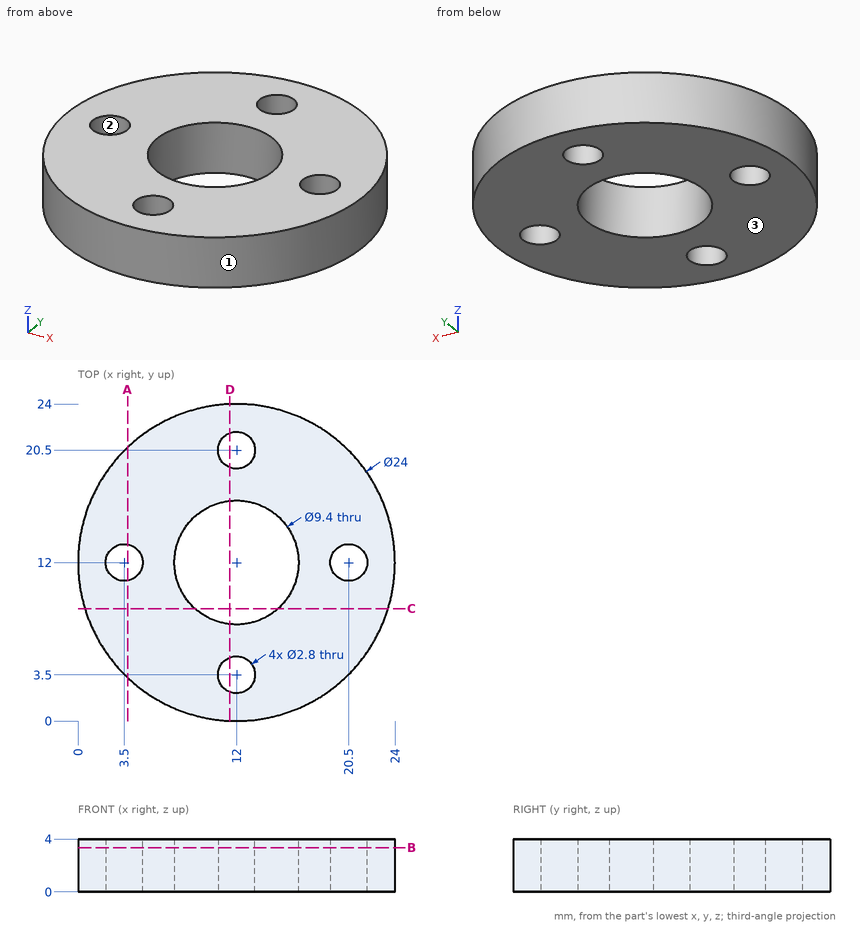
Could you check a few things on this drawing? It's one solid part, dimensions in mm from its lowest x, y, z. Round coordinates to 2 decimals unless told otherwise and drop trailing zeros. Order: outer loops, then holes, each group sorted by start corner. A loop starts at its lowest first (then second) coordinate and runs counter-clockwise, first axis right, second up. Notation, with made-up numbers: M 2.5,-6 L 7.5,-6 A6 cw 7.5,2 Z; hole C -29.5,18 d9. An arc over 180 degrees is marked long. Return JSON: item names as keys, results as strings. Group by question number.
1. If we section it at B-B on z = 3.35: List the corners of the cut face in (x, y) for me, then the cut area to 3 significant figures.
2. Please list where these lines run through material, in increasing order: probe 1 along Y at (x, z) = (12, 0.9); probe 2 along Y at (x, z) = (3.5, 2.4); probe 3 along Y at (x, z) = (15.25, 2.6).
3. If we mould it in two halves opening along X, with no side actions, what happens to the marked faces 1, 2 and 3? For each: pulls with the +X half, pulls with the -X half, needs draft (parallel to the pull), parting line crosses it, or undercut.
4. If we section it at C-C on y = 8.5: List the corners of the cut face in (x, z) for me, then the cut area to 3 significant figures.
5. If we section it at A-A on x = 3.75: List the corners of the cut face in (y, z) for me, then the cut area to 3 significant figures.
6. I'm going to push flat-ended pins straight in: pin 1 Ø3 at (x, y) = (20.5, 12) entering from +Z; pin 2 Ø1.5 at (x, z) = (3.5, 0.5) entering from -Y; pin 3 Ø1.5 at (y, z) = (18, 3.5) entering from +X; pin 4 Ø1.5 at (y, z) = (7, 3) entering from +X. Where does each tip first touch, or does it pass through?
7. If we section it at D-D on x = 11.5: List the corners of the cut face in (y, z) for me, then the cut area to 3 significant figures.
Reply:
{
 "1": {"outline": "C 12,12 d24; hole C 3.5,12 d2.8; hole C 12,12 d9.4; hole C 12,3.5 d2.8; hole C 12,20.5 d2.8; hole C 20.5,12 d2.8", "area": "358 mm^2"},
 "2": {"probe 1": "0 to 2.1, 4.9 to 7.3, 16.7 to 19.1, 21.9 to 24", "probe 2": "3.53 to 10.6, 13.4 to 20.47", "probe 3": "0.45 to 8.6, 15.4 to 23.55"},
 "3": {"face 1": "parting line crosses it", "face 2": "undercut", "face 3": "needs draft"},
 "4": {"outline": "M 0.52,0 L 8.86,0 L 8.86,4 L 0.52,4 Z; M 15.14,0 L 23.48,0 L 23.48,4 L 15.14,4 Z", "area": "66.7 mm^2"},
 "5": {"outline": "M 3.29,0 L 10.62,0 L 10.62,4 L 3.29,4 Z; M 13.38,0 L 20.71,0 L 20.71,4 L 13.38,4 Z", "area": "58.7 mm^2"},
 "6": {"pin 1": "z = 4", "pin 2": "y = 2.84", "pin 3": "x = 22.79", "pin 4": "x = 23.22"},
 "7": {"outline": "M 0.01,0 L 2.19,0 L 2.19,4 L 0.01,4 Z; M 4.81,0 L 7.33,0 L 7.33,4 L 4.81,4 Z; M 16.67,0 L 19.19,0 L 19.19,4 L 16.67,4 Z; M 21.81,0 L 23.99,0 L 23.99,4 L 21.81,4 Z", "area": "37.6 mm^2"}
}
